For this review, take the finished solid that the model builds, in its own axes (mm). A direction names the side the tool comes from. Give positions to 0.01 mm unless a question says otherwise; leave off trailing zeros. Loops run counter-clockwise (first coordinate to the right, second up) from the corner with the lowest first, then second, coordinate; pieces in that order, holes last. Notation, with made-up numbers: (83.25, 31) - (128.25, 31) arc R37 cw to (128.25, 68) - close; hole circle Ø3 at (18.25, 8). An arc over 180 degrees is marked (long way). Put each result on its own line as item: value. Start each with the question number.
from build123d import *

# Parameters (mm, degrees)
SKETCH_2_W                       = 75
SKETCH_2_H                       = 42
SM_BASE_FLANGE_1_DEPTH           = 2
SM_EDGE_FLANGE_1_STRIP_W         = 9.4732
SM_EDGE_FLANGE_1_STRIP_H         = 2
SM_EDGE_FLANGE_1_STRIP_CUT_DEPTH = 42
SM_EDGE_FLANGE_1_DEPTH           = 42
SM_EDGE_FLANGE_2_STRIP_W         = 9.4732
SM_EDGE_FLANGE_2_STRIP_H         = 2
SM_EDGE_FLANGE_2_STRIP_CUT_DEPTH = 42
SM_EDGE_FLANGE_2_DEPTH           = 42
SM_EDGE_FLANGE_3_STRIP_W         = 9.4732
SM_EDGE_FLANGE_3_STRIP_H         = 2
SM_EDGE_FLANGE_3_STRIP_CUT_DEPTH = 42
SM_EDGE_FLANGE_3_DEPTH           = 42
SM_EDGE_FLANGE_4_STRIP_W         = 9.4732
SM_EDGE_FLANGE_4_STRIP_H         = 2
SM_EDGE_FLANGE_4_STRIP_CUT_DEPTH = 42
SM_EDGE_FLANGE_4_DEPTH           = 42
HOLE_WIZARD_M2_4_AT_2_COUNT      = 2
HOLE_WIZARD_M2_4_AT_2_PITCH      = 36
HOLE_WIZARD_M2_4_AT_3_COUNT      = 2
HOLE_WIZARD_M2_4_AT_3_PITCH      = 85
HOLE_WIZARD_M2_4_AT_4_COUNT      = 2
HOLE_WIZARD_M2_4_AT_4_PITCH      = 92.309262807
SKETCH_27_W                      = 8.7366
SKETCH_27_H                      = 30
CUT_EXTRUDE_2319_DEPTH           = 38


# Sheet-metal steps are written as plain solids
with BuildPart() as part:
    # Sketch 2 → 基体-法兰1 (new body)
    with BuildSketch(Plane(origin=(0, 0, 0), x_dir=(1, 0, 0), z_dir=(0, 1, 0))):
        with Locations((21.966960091, -5.622610863)):
            Rectangle(SKETCH_2_W, SKETCH_2_H)
    extrude(amount=-SM_BASE_FLANGE_1_DEPTH)

    # 边线-法兰1 strip (across the edge) → 边线-法兰1 strip cut (cut)
    with BuildSketch(Plane(origin=(-15.533039909, -2, 26.622610863), x_dir=(1, 0, 0), z_dir=(0, 0, -1))):
        with Locations((-4, -1)):
            Rectangle(SM_EDGE_FLANGE_1_STRIP_W, SM_EDGE_FLANGE_1_STRIP_H)
    extrude(amount=SM_EDGE_FLANGE_1_STRIP_CUT_DEPTH, mode=Mode.SUBTRACT)

    # 边线-法兰1 section (across the edge) → 边线-法兰1 (add)
    with BuildSketch(Plane(origin=(-15.533039909, -2, 26.622610863), x_dir=(1, 0, 0), z_dir=(0, 0, -1))):
        with BuildLine():
            Line((-2, 0.7366), (-2, 30))
            Line((-2, 30), (0, 30))
            Line((0, 30), (0, 0.7366))
            ThreePointArc((0, 0.7366), (0.215745145, 0.215745145), (0.7366, 0))
            Line((0.7366, 0), (0.7366, -2))
            ThreePointArc((0.7366, -2), (-1.198468417, -1.198468417), (-2, 0.7366))
        make_face()
    extrude(amount=SM_EDGE_FLANGE_1_DEPTH)

    # 边线-法兰2 strip (across the edge) → 边线-法兰2 strip cut (cut)
    with BuildSketch(Plane(origin=(59.466960091, -2, -15.377389137), x_dir=(-1, 0, 0), z_dir=(0, 0, 1))):
        with Locations((-4, -1)):
            Rectangle(SM_EDGE_FLANGE_2_STRIP_W, SM_EDGE_FLANGE_2_STRIP_H)
    extrude(amount=SM_EDGE_FLANGE_2_STRIP_CUT_DEPTH, mode=Mode.SUBTRACT)

    # 边线-法兰2 section (across the edge) → 边线-法兰2 (add)
    with BuildSketch(Plane(origin=(59.466960091, -2, -15.377389137), x_dir=(-1, 0, 0), z_dir=(0, 0, 1))):
        with BuildLine():
            Line((-2, 0.7366), (-2, 30))
            Line((-2, 30), (0, 30))
            Line((0, 30), (0, 0.7366))
            ThreePointArc((0, 0.7366), (0.215745145, 0.215745145), (0.7366, 0))
            Line((0.7366, 0), (0.7366, -2))
            ThreePointArc((0.7366, -2), (-1.198468417, -1.198468417), (-2, 0.7366))
        make_face()
    extrude(amount=SM_EDGE_FLANGE_2_DEPTH)

    # 边线-法兰3 strip (across the edge) → 边线-法兰3 strip cut (cut)
    with BuildSketch(Plane(origin=(-17.533039909, -32, -15.377389137), x_dir=(0, 1, 0), z_dir=(0, 0, 1))):
        with Locations((-4, -1)):
            Rectangle(SM_EDGE_FLANGE_3_STRIP_W, SM_EDGE_FLANGE_3_STRIP_H)
    extrude(amount=SM_EDGE_FLANGE_3_STRIP_CUT_DEPTH, mode=Mode.SUBTRACT)

    # 边线-法兰3 section (across the edge) → 边线-法兰3 (add)
    with BuildSketch(Plane(origin=(-17.533039909, -32, -15.377389137), x_dir=(0, 1, 0), z_dir=(0, 0, 1))):
        with BuildLine():
            Line((-2, 0.7366), (-2, 6))
            Line((-2, 6), (0, 6))
            Line((0, 6), (0, 0.7366))
            ThreePointArc((0, 0.7366), (0.215745145, 0.215745145), (0.7366, 0))
            Line((0.7366, 0), (0.7366, -2))
            ThreePointArc((0.7366, -2), (-1.198468417, -1.198468417), (-2, 0.7366))
        make_face()
    extrude(amount=SM_EDGE_FLANGE_3_DEPTH)

    # 边线-法兰4 strip (across the edge) → 边线-法兰4 strip cut (cut)
    with BuildSketch(Plane(origin=(61.466960091, -32, 26.622610863), x_dir=(0, 1, 0), z_dir=(0, 0, -1))):
        with Locations((-4, -1)):
            Rectangle(SM_EDGE_FLANGE_4_STRIP_W, SM_EDGE_FLANGE_4_STRIP_H)
    extrude(amount=SM_EDGE_FLANGE_4_STRIP_CUT_DEPTH, mode=Mode.SUBTRACT)

    # 边线-法兰4 section (across the edge) → 边线-法兰4 (add)
    with BuildSketch(Plane(origin=(61.466960091, -32, 26.622610863), x_dir=(0, 1, 0), z_dir=(0, 0, -1))):
        with BuildLine():
            Line((-2, 0.7366), (-2, 6))
            Line((-2, 6), (0, 6))
            Line((0, 6), (0, 0.7366))
            ThreePointArc((0, 0.7366), (0.215745145, 0.215745145), (0.7366, 0))
            Line((0.7366, 0), (0.7366, -2))
            ThreePointArc((0.7366, -2), (-1.198468417, -1.198468417), (-2, 0.7366))
        make_face()
    extrude(amount=SM_EDGE_FLANGE_4_DEPTH)

    # 草图26 → M2*4 (revolve, cut)
    with BuildSketch(Plane(origin=(-20.533039909, -32, -12.377389137), x_dir=(0, 0, 1), z_dir=(1, 0, 0))):
        Polygon((0, 0), (0, 2), (1, 2), (1, 1), (2, 0), align=None)
    hole_wizard_m2_4 = revolve(axis=Axis((-20.533039909, -25.65, -12.377389137), (0, -1, 0)), mode=Mode.SUBTRACT)

    # M2*4 at 2: M2*4 ×2
    with Locations(*[(0, 0, i * HOLE_WIZARD_M2_4_AT_2_PITCH) for i in range(1, HOLE_WIZARD_M2_4_AT_2_COUNT)]):
        add(hole_wizard_m2_4, mode=Mode.SUBTRACT)

    # M2*4 at 3: M2*4 ×2
    with Locations(*[(i * HOLE_WIZARD_M2_4_AT_3_PITCH, 0, 0) for i in range(1, HOLE_WIZARD_M2_4_AT_3_COUNT)]):
        add(hole_wizard_m2_4, mode=Mode.SUBTRACT)

    # M2*4 at 4: M2*4 ×2
    with Locations(*[Vector(0.9208176667771376, 0, 0.38999336475266905) * (i * HOLE_WIZARD_M2_4_AT_4_PITCH) for i in range(1, HOLE_WIZARD_M2_4_AT_4_COUNT)]):
        add(hole_wizard_m2_4, mode=Mode.SUBTRACT)

    # 草图27 → Cut-Extrude 2319 (cut)
    with BuildSketch(Plane(origin=(0, 0, 0), x_dir=(1, 0, 0), z_dir=(0, 1, 0))):
        with Locations((-19.164739909, -5.622610863)):
            Rectangle(SKETCH_27_W, SKETCH_27_H)
        with Locations((63.098660091, -5.622610863)):
            Rectangle(SKETCH_27_W, SKETCH_27_H)
    extrude(amount=-CUT_EXTRUDE_2319_DEPTH, mode=Mode.SUBTRACT)


solid = part.part
1) Take a section at C-C on z = 17.5. State the section outline as (x, y) points, and give its area (3 significant figures).
2) Mouldability with a two-part tool opening along X and no side actions: class faces 1 (the flat face through (21, -2, 5)), 2 (the flat face through (67.467, -33, -12)), 3 (the flat face through (61, -19, 20.623)) as released by +X, released by -X, zero draft, split by the parting line, or undercut.
3) Machinability: for faces 4 (the cylindrical face through (-16.313, -33.177, 23.581)), 5 (the flat face through (-14.796, -1, 6)), 6 (the flat face through (-23, -32, -12)), 7 (the flat face through (67, -32, 24)), which of the approach directions +Z, -Z, +X, -X, +Y, -Y give a long, thin tool a straight path to every point of the face, cutting with its end or side? Answer none if there is none.
4) Take a section at B-B on x = 39. State the section outline as (y, z) points.
5) Take a section at A-A on y = -20. State the section outline as (x, z) points, and give its area (3 significant figures).
6) Insertion check: P1, Ø1.8, axis at x = -20.53, z = -12.38, coming from the +Y side; P2, Ø1.8, axis at y = -12.5, z = 24.5, coming from the -X side; P3, Ø6.5, axis at y = -24, z = 22.5, coming from the +X side; P4, Ø12.5, axis at x = 5, z = 0, coming from the -Y side. Each pin has a flat end and moves straight along its axis. Give the tip position at first contact, or say it passes through.
7) Wall thickness on probe 1 along X at (y, z) = (-22, 21); probe 2 along Z at (x, y) = (-17.5, -18.5); probe 3 along Y at (x, z) = (31.5, -11.5): over which ranges is each line inside the solid? List them lowest first.
Answers follow:
1. outline: (-14.8, -2) - (58.73, -2) - (58.73, 0) - (-14.8, 0) - close
1. area: 147 mm2
2. face 1: undercut
2. face 2: released by +X
2. face 3: zero draft
3. face 4: +Z, -Z, -Y
3. face 5: -X, +Y, -Y
3. face 6: +Z, -Z, -X, +Y
3. face 7: +Z, -Z, +X, +Y
4. outline: (-2, -15.38) - (0, -15.38) - (0, 26.62) - (-2, 26.62) - close
5. outline: (-17.53, -15.38) - (-15.53, -15.38) - (-15.53, -9.38) - (-17.53, -9.38) - close; (-17.53, 20.62) - (-15.53, 20.62) - (-15.53, 26.62) - (-17.53, 26.62) - close; (59.47, -15.38) - (61.47, -15.38) - (61.47, -9.38) - (59.47, -9.38) - close; (59.47, 20.62) - (61.47, 20.62) - (61.47, 26.62) - (59.47, 26.62) - close
5. area: 48.0 mm2
6. P1: through
6. P2: x = -17.53
6. P3: x = 61.47
6. P4: y = -2
7. probe 1: -17.53 to -15.53, 59.47 to 61.47
7. probe 2: -15.38 to -9.38, 20.62 to 26.62
7. probe 3: -2 to 0
